Answer from the drawing. Dimensions are ordinates in mm from the lowest x, y and z of the part. Coordinates: 2 decimals unless noted, no trailing zeros. Order: outer loops, then holes, each group sorted by start corner. A loop starts at its lowest first (then second) coordinate and runs counter-clockwise, first axis right, second up. Notation, with made-up numbers: (43, 78.5) -> (51, 78.5) arc R11 cw to (51, 93.5) -> close; hole circle Ø4 at (-9.75, 27.25). An arc over 180 degrees is marked (long way). Answer as a JSON object with one key per item and string values. Group by question number.
1) Section C-C on y = 42 is taken. Determine the outline of the cut face in (x, z) (1 decimal).
2) Section A-A on y = 18 is taken. Determine the outline of the cut face in (x, z).
3) Given pin 1 (5 mm diameter, centred on y = 19.42, z = 9.35, fed in from +X), flat-ended and moving along its own axis, determine where the tip first touches the part or whether it passes through.
4) Section B-B on z = 41 is taken. Determine the outline of the cut face in (x, y) (1 decimal).
5) Section D-D on x = 2.4 is taken. Count the separate pieces of the cut face and the enclosed holes in it, and give its area (3 significant figures).
6) Consider L1, parallel to Z at x = 2.45, y = 21.5 (1 decimal); L2, parallel to Y at x = 2.95, z = 21.5 (1 decimal); L3, parallel to Z at x = 2, y = 27 (1 decimal). Determine where each line is inside the solid, lowest interval first.
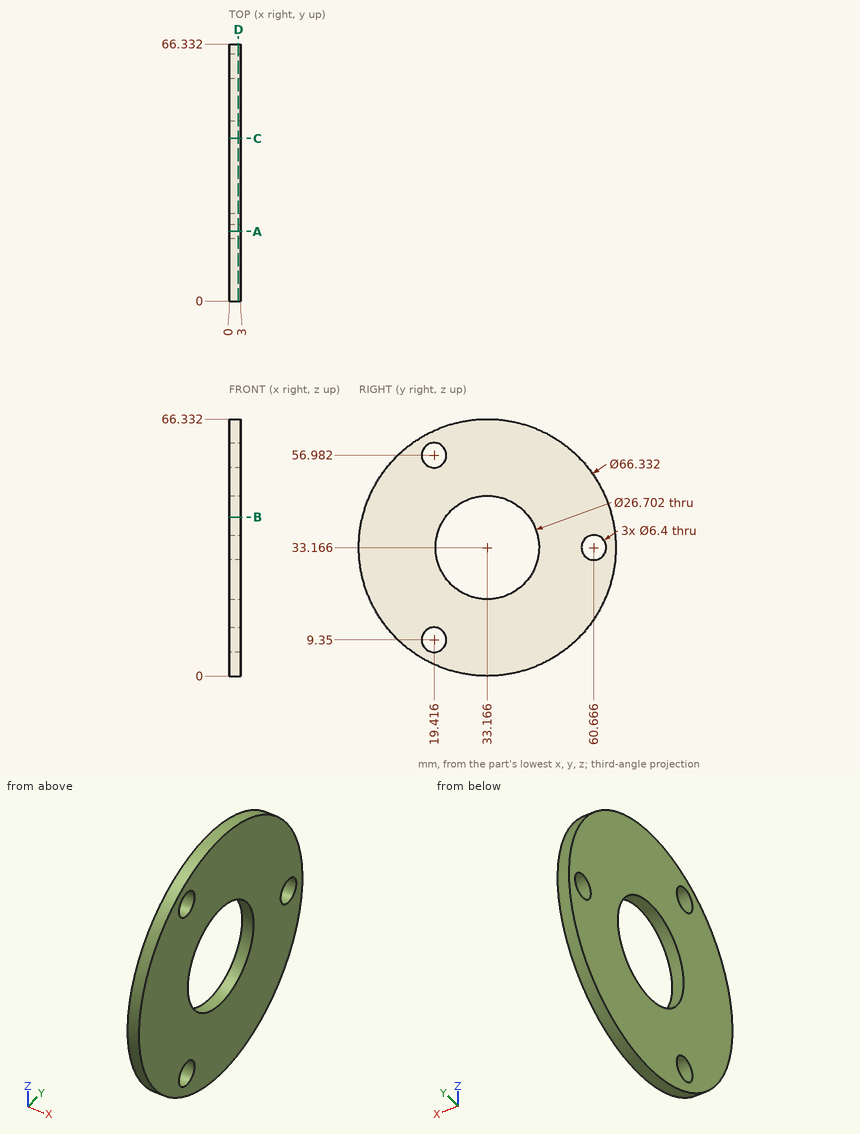
Worked answers:
{
 "1": {"outline": "(0, 1.2) -> (3, 1.2) -> (3, 23.2) -> (0, 23.2) -> close; (0, 43.2) -> (3, 43.2) -> (3, 65.1) -> (0, 65.1) -> close"},
 "2": {"outline": "(0, 3.67) -> (3, 3.67) -> (3, 6.48) -> (0, 6.48) -> close; (0, 12.22) -> (3, 12.22) -> (3, 54.11) -> (0, 54.11) -> close; (0, 59.85) -> (3, 59.85) -> (3, 62.66) -> (0, 62.66) -> close"},
 "3": {"pin 1": "passes through"},
 "4": {"outline": "(0, 0.9) -> (3, 0.9) -> (3, 22.4) -> (0, 22.4) -> close; (0, 44) -> (3, 44) -> (3, 65.4) -> (0, 65.4) -> close"},
 "5": {"separate pieces": "1", "enclosed holes": "4", "area": "2,800 mm²"},
 "6": {"L1": "z = 2.1 to 6.9, 11.8 to 26.7, 39.7 to 54.6, 59.4 to 64.2", "L2": "y = 2.1 to 26.7, 39.7 to 64.2", "L3": "z = 0.6 to 21.3, 45 to 65.8"}
}
